Verification items for the finished model (mm, model axes). A direction names the side the tool comes from. Give positions to 0.01 mm unless a question says otherwise; leave off trailing zeros. Write each loop counter-clockwise with the first axis right and the second up, starting at its lowest first coordinate (ties: lowest second). Pieces come first, ordered by that corner, then holes. Notation, with made-up numbers: M 22,-16.5 L 26,-16.5 A19 cw 26,-0.5 Z; hole C -22,32 d8. An arc over 180 degrees is marked long. Answer as a JSON object with one key per item and string values.
```python
from build123d import *

# Parameters (mm, degrees)
SKETCH1_W                = 20
SKETCH1_H                = 15
BOSS_EXTRUDE1_DEPTH      = 18
SKETCH2_W                = 12
SKETCH2_H                = 8
BOSS_EXTRUDE2_DEPTH      = 5
SKETCH4_W                = 4
SKETCH4_H                = 4
BOSS_EXTRUDE4_DEPTH      = 0.5
SKETCH3_W                = 3.5
SKETCH3_H                = 8
BOSS_EXTRUDE3_DEPTH      = 4
SKETCH5_W                = 4.004840827
SKETCH5_H                = 3.775181513
SKETCH5_W_2              = 3.995159173
SKETCH5_W_3              = 3.9
BOSS_EXTRUDE5_DEPTH      = 0.5
BOSS_EXTRUDE6_DEPTH      = 2
BOSS_EXTRUDE6_DEPTH_BACK = 43
SKETCH7_W                = 18
SKETCH7_H                = 20
FRONT_START              = 13
SKETCH8_W                = 7
SKETCH8_H                = 7
FRONT_PAWS_DEPTH         = 33
BOSS_EXTRUDE8_DEPTH      = 18
BOSS_EXTRUDE9_START      = -5
SKETCH10_W               = 7
SKETCH10_H               = 7
BOSS_EXTRUDE9_DEPTH      = 20
CHAMFER1_SIZE            = 5
CHAMFER1_SIZE2           = 7.071067812
BOSS_EXTRUDE10_START     = -37
SKETCH11_W               = 4
SKETCH11_H               = 4
BOSS_EXTRUDE10_DEPTH     = 30
SKETCH13_W               = 4
SKETCH13_H               = 4
BOSS_EXTRUDE11_DEPTH     = 30


with BuildPart() as part:
    # Sketch1 → Boss-Extrude1 (new body)
    with BuildSketch(Plane(origin=(0, 0, 0), x_dir=(1, 0, 0), z_dir=(0, 1, 0))):
        Rectangle(SKETCH1_W, SKETCH1_H)
    extrude(amount=BOSS_EXTRUDE1_DEPTH)

    # Sketch2 → Boss-Extrude2 (add)
    with BuildSketch(Plane(origin=(0, 18, 0), x_dir=(1, 0, 0), z_dir=(0, 1, 0))):
        with Locations((0, -3.5)):
            Rectangle(SKETCH2_W, SKETCH2_H)
    extrude(amount=BOSS_EXTRUDE2_DEPTH)

    # Sketch4 → Boss-Extrude4 (add)
    with BuildSketch(Plane(origin=(0, 23, 0), x_dir=(1, 0, 0), z_dir=(0, 1, 0))):
        with Locations((0.004840827, -1.5)):
            Rectangle(SKETCH4_W, SKETCH4_H)
    extrude(amount=BOSS_EXTRUDE4_DEPTH)

    # Sketch3 → Boss-Extrude3 (add)
    with BuildSketch(Plane(origin=(0, 0, -7.5), x_dir=(-1, 0, 0), z_dir=(0, 0, -1))):
        with Locations((-4.75, 4)):
            Rectangle(SKETCH3_W, SKETCH3_H)
        with Locations((4.75, 4)):
            Rectangle(SKETCH3_W, SKETCH3_H)
    extrude(amount=BOSS_EXTRUDE3_DEPTH)

    # Sketch5 → Boss-Extrude5 (add)
    with BuildSketch(Plane(origin=(0, 18, 0), x_dir=(1, 0, 0), z_dir=(0, 1, 0))):
        with Locations((-3.997579587, 2.387590757)):
            Rectangle(SKETCH5_W, SKETCH5_H)
        with Locations((4.002420414, 2.387590757)):
            Rectangle(SKETCH5_W_2, SKETCH5_H)
        with Locations((-8.05, 2.387590757)):
            Rectangle(SKETCH5_W_3, SKETCH5_H)
        with Locations((8.05, 2.387590757)):
            Rectangle(SKETCH5_W_3, SKETCH5_H)
    extrude(amount=BOSS_EXTRUDE5_DEPTH)

    # Sketch7 → Boss-Extrude6 (add, two sides: drawn at the far end of the back side and taken through both)
    with BuildSketch(Plane(origin=(0, -3.75, 3.75), x_dir=(1, 0, 0), z_dir=(0, 0.7071067811865488, -0.7071067811865464)).offset(-BOSS_EXTRUDE6_DEPTH_BACK)):
        with Locations((0, -5.303300859)):
            Rectangle(SKETCH7_W, SKETCH7_H)
    extrude(amount=BOSS_EXTRUDE6_DEPTH + BOSS_EXTRUDE6_DEPTH_BACK)

    # Sketch8 → front paws (add)
    with BuildSketch(Plane.XY.offset(FRONT_START)):
        with Locations((-6.458894343, 3.691922456)):
            Rectangle(SKETCH8_W, SKETCH8_H)
        with Locations((6.458894343, 3.691922456)):
            Rectangle(SKETCH8_W, SKETCH8_H)
    extrude(amount=FRONT_PAWS_DEPTH)

    # Sketch9 → Boss-Extrude8 (add)
    with BuildSketch(Plane(origin=(9, 0, 0), x_dir=(0, 0, -1), z_dir=(1, 0, 0))):
        Polygon((-44.976659403, -23.334523779), (-30.834523779, -37.476659403), (-44.976659403, -51.618795027), align=None)
    extrude(amount=-BOSS_EXTRUDE8_DEPTH)

    # Sketch10 → Boss-Extrude9 (add)
    with BuildSketch(Plane(origin=(0, 0, 0), x_dir=(1, 0, 0), z_dir=(0, 1, 0)).offset(BOSS_EXTRUDE9_START)):
        with Locations((-6.458894343, -41.986772092)):
            Rectangle(SKETCH10_W, SKETCH10_H)
        with Locations((6.458894343, -41.986772092)):
            Rectangle(SKETCH10_W, SKETCH10_H)
    extrude(amount=-BOSS_EXTRUDE9_DEPTH)

    # Chamfer1
    chamfer1_edges = [part.edges().sort_by_distance(p)[0] for p in [
        (0, -51.618795027, 44.976659403),
    ]]
    chamfer1_side = [part.faces().sort_by_distance(p)[0] for p in [
        (0, -28.637824638, 21.995689014),
    ]]
    chamfer(chamfer1_edges, length=CHAMFER1_SIZE, length2=CHAMFER1_SIZE2, reference=chamfer1_side[0])

    # Sketch11 → Boss-Extrude10 (add)
    with BuildSketch(Plane(origin=(0, 0, 0), x_dir=(1, 0, 0), z_dir=(0, 1, 0)).offset(BOSS_EXTRUDE10_START)):
        with Locations((0, -40.063214372)):
            Rectangle(SKETCH11_W, SKETCH11_H)
    extrude(amount=-BOSS_EXTRUDE10_DEPTH)

    # Sketch13 → Boss-Extrude11 (add)
    with BuildSketch(Plane(origin=(0, -12.468392814, -12.468392814), x_dir=(-1, 0, 0), z_dir=(0, -0.7071067811865465, -0.7071067811865487))):
        with Locations((0, -75.119338461)):
            Rectangle(SKETCH13_W, SKETCH13_H)
    extrude(amount=BOSS_EXTRUDE11_DEPTH)


solid = part.part
```
1) Section check A-A on x = 4.75. Record the boundary of the cut face in (y, z), and give its area (3 significant figures).
Completed:
{"outline": "M -48.08,41.44 L -5.66,-0.99 L 0,4.67 L 0,-11.5 L 8,-11.5 L 8,-7.5 L 18,-7.5 L 18,-4.28 L 18.5,-4.28 L 18.5,-0.5 L 23,-0.5 L 23,7.5 L 2.83,7.5 L 8.49,13.16 L 7.19,14.45 L 7.19,46 L 0.19,46 L 0.19,21.45 L -16.84,38.49 L -5,38.49 L -5,45.49 L -25,45.49 L -25,44.98 L -44.55,44.98 Z", "area": "1,730 mm2"}
2) Access from +Z, -Z, +X, -X, +Y, -Y to the whole of each face (thin tool, end or side, straight path). Record for faces 1 (the face through (6.5, 4, -9)), 2 (the face through (6, -5, 42)), 3 (the face through (-0.13, -2.87, 1.8)), 4 (the face through (-6.5, 4, -9)).
Completed:
{"face 1": "-Z, +X, +Y, -Y", "face 2": "+Z, +X, -X", "face 3": "-Z, +X, -X", "face 4": "-Z, -X, +Y, -Y"}
3) Section check B-B on y = -21.5. Record the boundary of the cut face in (x, z), and give its area (3 significant figures).
Completed:
{"outline": "M -9.96,38.49 L -9,38.49 L -9,14.86 L 9,14.86 L 9,38.49 L 9.96,38.49 L 9.96,45.49 L 2.96,45.49 L 2.96,43.14 L -2.96,43.14 L -2.96,45.49 L -9.96,45.49 Z", "area": "551 mm2"}
4) Section check C-C on y = 12. Record the boundary of the cut face in (x, z), and give its area (3 significant figures).
Completed:
{"outline": "M -10,-7.5 L 10,-7.5 L 10,7.5 L -10,7.5 Z", "area": "300 mm2"}
5) Section check D-D on y = -63. Record the boundary of the cut face in (x, z), and give its area (3 significant figures).
Completed:
{"outline": "M -2,38.06 L 2,38.06 L 2,42.06 L -2,42.06 Z", "area": "16.0 mm2"}
6) Go/stop test with flat-tipped pins: pin 1 (5.5 mm diameter, centred on x = -5, y = -14.5, fed in from +Z); pin 2 (3.5 mm diameter, centred on y = -17, z = 43.5, fed in from +X); pin 3 (5.5 mm diameter, centred on x = 7.5, y = -19.5, fed in from -Z). Record where each tip stops, or that it passes through.
Completed:
{"pin 1": "stops at z = 45.49", "pin 2": "stops at x = 9.96", "pin 3": "stops at z = 10.11"}
7) Thickness scan on L1, parallel to Y at x = 9.25, z = 22.5; L2, parallel to Z at x = 3.75, y = 9; L3, parallel to X at y = -33, z = 43.5. Record the ranges inside material, lowest first.
Completed:
{"L1": "y = 0.19 to 7.19", "L2": "z = -7.5 to 7.5", "L3": "x = -9 to 9"}
8) Release check for a two-part mould opening along Z. For faces 5 (the face through (0, -57, 42.063)), 6 (the face through (9.959, 4, 29)), 7 (the face through (0, 11, 7.5)) record: pulls with the +Z half, pulls with the -Z half, needs draft (parallel to the pull), parting line crosses it, or undercut.
Completed:
{"face 5": "pulls with the +Z half", "face 6": "needs draft", "face 7": "undercut"}
